from build123d import *

# Parameters (mm, degrees)
SKETCH1_R           = 1.75
BOSS_EXTRUDE1_DEPTH = 2.4
BOSS_EXTRUDE2_DEPTH = 57.4
SKETCH3_W           = 30
SKETCH3_H           = 10.390128061
BOSS_EXTRUDE3_DEPTH = 2.4
FILLET1_START       = -61.5000001
FILLET1_DEPTH       = 23.0000001
FILLET1_START_2     = 2.4
FILLET1_2_DEPTH     = 7.99015084
FILLET2_R           = 2.4


with BuildPart() as part:
    # Sketch1 → Boss-Extrude1 (new body)
    with BuildSketch(Plane(origin=(0, 0, 0), x_dir=(1, 0, 0), z_dir=(0, 1, 0))):
        with BuildLine():
            Line((-44.25, 50), (-44.25, 20.75))
            ThreePointArc((-44.25, 20.75), (-42.565863992, 16.684136008), (-38.5, 15))
            Line((-38.5, 15), (-15, 15))
            Line((-15, 15), (-15, -15))
            Line((-15, -15), (-38.5, -15))
            ThreePointArc((-38.5, -15), (-42.565863992, -16.684136008), (-44.25, -20.75))
            Line((-44.25, -20.75), (-44.25, -50))
            ThreePointArc((-44.25, -50), (-50, -55.75), (-55.75, -50))
            Line((-55.75, -50), (-55.75, -20.75))
            ThreePointArc((-55.75, -20.75), (-57.434136008, -16.684136008), (-61.5, -15))
            Line((-61.5, -15), (-72.4, -15))
            Line((-72.4, -15), (-72.4, 15))
            Line((-72.4, 15), (-61.5, 15))
            ThreePointArc((-61.5, 15), (-57.434136008, 16.684136008), (-55.75, 20.75))
            Line((-55.75, 20.75), (-55.75, 50))
            ThreePointArc((-55.75, 50), (-50, 55.75), (-44.25, 50))
        make_face()
        with Locations(Location((-50, 50, 0), (0, 0, 270))):
            Circle(SKETCH1_R, mode=Mode.SUBTRACT)
        with Locations(Location((-50, -50, 0), (0, 0, 270))):
            Circle(SKETCH1_R, mode=Mode.SUBTRACT)
    extrude(amount=BOSS_EXTRUDE1_DEPTH)

    # Sketch2 → Boss-Extrude2 (add)
    with BuildSketch(Plane(origin=(-15, 0, 0), x_dir=(0, 0, -1), z_dir=(1, 0, 0))):
        Polygon((-15, 0), (-15, 10.390128061), (-7.490128061, 10.390128061), (-0.5, 3.4), (-0.5, 2.4), (0.5, 2.4), (0.5, 3.4), (7.490128061, 10.390128061), (15, 10.390128061), (15, 0), align=None)
    extrude(amount=-BOSS_EXTRUDE2_DEPTH)

    # Sketch3 → Boss-Extrude3 (add)
    with BuildSketch(Plane.ZY.offset(72.4)):
        with Locations((0, 5.195064031)):
            Rectangle(SKETCH3_W, SKETCH3_H)
    extrude(amount=-BOSS_EXTRUDE3_DEPTH)

    # Fillet1: read off the stored shape, not the designer's step
    # Fillet1 outline → Fillet1 (add)
    with BuildSketch(Plane.YZ.offset(FILLET1_START)):
        with BuildLine():
            Line((2.4, -15), (2.4, -30.992591285))
            ThreePointArc((2.4, -30.992591285), (4.508703468, -22.053826918), (10.39015084, -14.999982893))
            Line((10.39015084, -14.999982893), (2.4, -15))
        make_face()
        with BuildLine():
            ThreePointArc((10.39015084, 14.999982893), (4.508703468, 22.053826918), (2.4, 30.992591285))
            Line((2.4, 30.992591285), (2.4, 15))
            Line((2.4, 15), (10.39015084, 14.999982893))
        make_face()
    extrude(amount=FILLET1_DEPTH)

    # Fillet1 2 outline → Fillet1 2 (cut)
    with BuildSketch(Plane(origin=(0, 0, 0), x_dir=(1, 0, 0), z_dir=(0, 1, 0)).offset(FILLET1_START_2)):
        with BuildLine():
            ThreePointArc((-38.5, -15), (-42.565863992, -16.684136008), (-44.25, -20.75))
            Line((-44.25, -20.75), (-44.25, -32))
            Line((-44.25, -32), (-38.5, -32))
            Line((-38.5, -32), (-38.5, -15))
        make_face()
        with BuildLine():
            Line((-61.5000001, -32), (-55.75, -32))
            Line((-55.75, -32), (-55.75, -20.75))
            ThreePointArc((-55.75, -20.75), (-57.434136008, -16.684136008), (-61.5, -15))
            Line((-61.5, -15), (-61.5000001, -32))
        make_face()
        with BuildLine():
            Line((-38.5, 15), (-38.5, 32))
            Line((-38.5, 32), (-44.25, 32))
            Line((-44.25, 32), (-44.25, 20.75))
            ThreePointArc((-44.25, 20.75), (-42.565863992, 16.684136008), (-38.5, 15))
        make_face()
        with BuildLine():
            Line((-55.75, 32), (-61.5000001, 32))
            Line((-61.5000001, 32), (-61.5, 15))
            ThreePointArc((-61.5, 15), (-57.434136008, 16.684136008), (-55.75, 20.75))
            Line((-55.75, 20.75), (-55.75, 32))
        make_face()
    extrude(amount=FILLET1_2_DEPTH, mode=Mode.SUBTRACT)

    # Fillet2
    fillet2_edges = [part.edges().sort_by_distance(p)[0] for p in [
        (-72.4, 5.19506403, 15),
        (-72.4, 5.19506403, -15),
        (-15, 5.19506403, -15),
        (-15, 5.19506403, 15),
    ]]
    fillet(fillet2_edges, radius=FILLET2_R)


solid = part.part
Source: CAD feature listing. Evaluate the final solid. Frame: model axes, mm. A direction names the side the tool comes from. Give positions to 0.01 mm unless a question says otherwise; leave off trailing zeros. Loops run counter-clockwise (first coordinate to the right, second up) from the corner with the lowest first, then second, coordinate; pieces in that order, holes last. Notation, with made-up numbers: (65, 89.5) -> (110, 89.5) arc R21 cw to (110, 102.5) -> close; hole circle Ø9 at (55, 70). An arc over 180 degrees is marked (long way). Use a Markdown table: item, result. Add a question column.
1) Section query D-D, the plane y = 7.5. Return the cut outline in (x, z).
2) First-contact query: pin 1 (0.5 mm diameter, centred on x = -45, y = 2.5, fed in from -Z); pin 2 (1.5 mm diameter, centred on y = 3, z = -26.5, fed in from +X); pin 3 (2.5 mm diameter, centred on x = -63.5, y = 7.5, fed in from +Z); pin 4 (1.6 mm diameter, centred on y = 4, z = -30, fed in from -X). Flat tips, straight axial feed; report the tip coordinate or a pass-through.
3) Section query B-B, the plane x = -36.5. Return the cut outline in (y, z).
4) Pull-direction query (Z, two-part tool) for faces 1 (the face through (-70, 7, 0)), 2 (the face through (-44.25, 1, -36)), 3 (the face through (-71.678, 5.122, 14.316)), 4 (the face through (-42.1, 6.8, -3.9)); classes: +Z half, -Z half, draft (parallel to the pull), parting line (faces both ways), or undercut.
5) Section query A-A, the plane y = 1.25. Return the cut outline in (x, z).
6) Line query: line 1 along X through (y, z) = (1.4, 50); line 2 along Y through (x, z) = (-46, 44). Output: solid intervals per line, ascending. Write a range as [from, to].
7) Reachability of faces 5 (the face through (-66, 5, 15)), 6 (the face through (-66, 5, -15)), 7 (the face through (-43, 10.39, 10)), 8 (the face through (-44.25, 1, 32)), 9 (the face through (-50.16, 4.45, -22.17)) from +Z, -Z, +X, -X, +Y, -Y: full face, straight path, thin tool, end or side. Return the list, or none.
8) Section query C-C, the plane z = 45. Return the cut outline in (x, y).
Numbers:
| question | item | result |
|---|---|---|
| 1 | outline | (-72.4, -12.6) arc R2.4 ccw to (-70, -15) -> (-61.5, -15) arc R5.75 cw to (-56.66, -17.65) -> (-43.34, -17.65) arc R5.75 cw to (-38.5, -15) -> (-17.4, -15) arc R2.4 ccw to (-15, -12.6) -> (-15, -4.6) -> (-70, -4.6) -> (-70, 4.6) -> (-15, 4.6) -> (-15, 12.6) arc R2.4 ccw to (-17.4, 15) -> (-38.5, 15) arc R5.75 cw to (-43.34, 17.65) -> (-56.66, 17.65) arc R5.75 cw to (-61.5, 15) -> (-70, 15) arc R2.4 ccw to (-72.4, 12.6) -> close |
| 2 | pin 1 | stops at z = -53.21 |
| 2 | pin 2 | stops at x = -44.25 |
| 2 | pin 3 | stops at z = 15 |
| 2 | pin 4 | passes through |
| 3 | outline | (0, -15) -> (10.39, -15) -> (10.39, -7.49) -> (3.4, -0.5) -> (2.4, -0.5) -> (2.4, 0.5) -> (3.4, 0.5) -> (10.39, 7.49) -> (10.39, 15) -> (0, 15) -> close |
| 4 | face 1 | undercut |
| 4 | face 2 | draft |
| 4 | face 3 | +Z half |
| 4 | face 4 | undercut |
| 5 | outline | (-72.4, -12.6) arc R2.4 ccw to (-70, -15) -> (-61.5, -15) arc R5.75 cw to (-55.75, -20.75) -> (-55.75, -50) arc R5.75 ccw to (-44.25, -50) -> (-44.25, -20.75) arc R5.75 cw to (-38.5, -15) -> (-17.4, -15) arc R2.4 ccw to (-15, -12.6) -> (-15, 12.6) arc R2.4 ccw to (-17.4, 15) -> (-38.5, 15) arc R5.75 cw to (-44.25, 20.75) -> (-44.25, 50) arc R5.75 ccw to (-55.75, 50) -> (-55.75, 20.75) arc R5.75 cw to (-61.5, 15) -> (-70, 15) arc R2.4 ccw to (-72.4, 12.6) -> close; hole circle Ø3.5 at (-50, -50); hole circle Ø3.5 at (-50, 50) |
| 6 | line 1 | x = [-55.75, -51.75], [-48.25, -44.25] |
| 6 | line 2 | y = [0, 2.4] |
| 7 | face 5 | +Z, -X, +Y, -Y |
| 7 | face 6 | -Z, -X, +Y, -Y |
| 7 | face 7 | +Z, -Z, +X, -X, +Y |
| 7 | face 8 | +Z, +X, +Y, -Y |
| 7 | face 9 | -Z, +X, -X, +Y |
| 8 | outline | (-55.75, 0) -> (-44.25, 0) -> (-44.25, 2.4) -> (-55.75, 2.4) -> close |
